Autodesk Inventor part; units mm, degrees
ref_plane "YZ Plane" through (0, 0, 0) normal (1, 0, 0) x (0, 1, 0)
ref_plane "XZ Plane" through (0, 0, 0) normal (0, 1, 0) x (-1, 0, 0)
ref_plane "XY Plane" through (0, 0, 0) normal (0, 0, 1) x (1, 0, 0)
sketch "Skizze1" plane through (0, 0, 0) normal (0, 1, 0) x (-1, 0, 0)
  circle A0 centre (0, 0) radius 25
  dimension "d0" = 50
extrude "Extrusion1" add sketch "Skizze1" along normal blind 20
sketch "Skizze2" plane through (0, 0, 0) normal (0, -1, 0) x (1, 0, 0)
  line L0 (-25, 25) -> (25, 25)
  line L1 (25, 25) -> (25, -25)
  line L2 (25, -25) -> (-25, -25)
  line L3 (-25, -25) -> (-25, 25)
  circle A0 centre (0, 0) radius 25
extrude "Extrusion2" add sketch "Skizze2" along normal blind 10
sketch "Skizze3" plane through (0, -10, 0) normal (0, -1, 0) x (1, 0, 0)
  circle A0 centre (0, 0) radius 5
  dimension "d5" = 10
extrude "Extrusion3" cut sketch "Skizze3" against normal up to next
properties part number "2ExtrusionenMitLoch"
Source: CAD feature listing. Evaluate the final solid. Frame: model axes, mm. A direction names the side the tool comes from. Coordinates: 2 decimals unless noted, no trailing zeros. Order: outer loops, then holes, each group sorted by start corner. A loop starts at its lowest first (then second) coordinate and runs counter-clockwise, first axis right, second up. Notation, with made-up numbers: M 28,-2.5 L 40,-2.5 A11 ccw 40,8.5 Z; hole C 69.25,76.5 d4. An arc over 180 degrees is marked long. Write each question's results on one line, items separated by ' | '. Start each with the question number.
1. Reachability of faces 1 (the face through (-20, 0, 19)), 2 (the face through (20, 0, -20)), 3 (the face through (-20, 0, -19)) from +Z, -Z, +X, -X, +Y, -Y: full face, straight path, thin tool, end or side. Return the list, or none.
2. Material intervals for L1, parallel to Z at x = 0, y = 2.25; L2, parallel to Z at x = 2, y = -5.5; L3, parallel to X at y = -7.5, z = 3.5, sorted ascending.
3. Draft query along X for faces 4 (the face through (-25, -5, 0)), 5 (the face through (-1.08, 4.79, -4.88)), 6 (the face through (-23.846, 9.86, -7.509)), 7 (the face through (0, -5, -25)). Return one class per face: +X half, -X half, draft (parallel to the pull), parting line (faces both ways), or undercut.
4. Section D-D, the plane z = 3. Return the cut outline in (x, y).
5. Section C-C, the plane y = -6.75. Return the cut outline in (x, z), then the cut area to 3 significant figures.
6. Section B-B, the plane x = -15. Return the cut outline in (y, z), then the cut area to 3 significant figures.
7. Pin query (flat end, axial travel): pin 1 (12 mm diameter, centred on y = 6.5, z = -6.5, fed in from +X) (3 decimals); pin 2 (1.5 mm diameter, centred on x = -18, y = 9, fed in from -Z); pin 3 (6 mm diameter, centred on x = 15, y = 11, fed in from +Z); pin 4 (8 mm diameter, centred on x = 0, z = 0, fed in from +Y). Return the tip coordinate at first contact, or that it passes through.
Solution:
1) face 1: +Z, -X, +Y | face 2: -Z, +X, +Y | face 3: -Z, -X, +Y
2) L1: -25 to -5, 5 to 25 | L2: -25 to -4.58, 4.58 to 25 | L3: -25 to -3.57, 3.57 to 25
3) face 4: -X half | face 5: undercut | face 6: parting line | face 7: draft
4) outline: M -25,-10 L -4,-10 L -4,20 L -24.82,20 L -24.82,0 L -25,0 Z; M 4,-10 L 25,-10 L 25,0 L 24.82,0 L 24.82,20 L 4,20 Z
5) outline: M -25,-25 L 25,-25 L 25,25 L -25,25 Z; hole C 0,0 d10 | area: 2,420 mm²
6) outline: M -10,-25 L 0,-25 L 0,-20 L 20,-20 L 20,20 L 0,20 L 0,25 L -10,25 Z | area: 1,300 mm²
7) pin 1: x = 24.995 | pin 2: z = -18.1 | pin 3: z = 21.93 | pin 4: through
